Part model, mm, in its own coordinate system. A direction names the side the tool comes from. Give positions to 0.01 mm unless a question says otherwise; leave off trailing zeros. Write each loop counter-clockwise with the first axis right and the second up, starting at its lowest first coordinate (ties: lowest second). Pieces come first, ordered by that corner, then holes. Notation, with made-up numbers: (13.25, -3.5) - (61.25, -3.5) arc R23 ccw to (61.25, 12.5) - close; hole circle Ø5 at (70.5, 10). An arc over 180 degrees is marked (long way). Answer in a Markdown table with one row per item. Add a question column.
1. Which spindle directions (+Z, -Z, +X, -X, +Y, -Y) get a long thin tool onto all of the face, cutting with end or side? Do faces 1 (the flat face through (-1, 20, 14)), 2 (the flat face through (41, 1.75, 18)), 3 (the flat face through (-1, 22.5, 13)). Say none if no direction does.
2. Band-saw the part on B-B on x = 32.25. Write the cut outline in (y, z).
3. Probe line 1 along Y through (x, z) = (-23.5, 9); line 2 along X through (y, z) = (11.5, 20.75); line 3 along Y through (x, z) = (32.25, 1.6). List the from-to ranges inside material, lowest first.
4. Band-saw the part on C-C on y = 0. Write the cut outline in (x, z) (3 decimals).
5. Drop a flat-ended pin along its axis: pin 1 Ø8 at (x, y) = (24, -4) entering from +Z. Give the stop position or say it passes through.
6. Band-saw the part on A-A on z = 18. State how many separate pieces and enclosed holes the cut face has, plus the area to 3 significant figures.
7. Pull direction X, two halves, no side cores. Call faces 4 (the flat face through (-1.75, 21, 18)), 5 (the cylindrical face through (41.9, 21.93, 12.82)), 6 (the flat face through (-42.5, 0, 13)): released by +X, released by -X, zero draft, split by the parting line, or undercut.
8. Band-saw the part on D-D on z = 12. Write the cut outline in (x, y), plus the area to 3 significant figures.
```python
from build123d import *

# Parameters (mm, degrees)
F0_W      = 85
F0_H      = 45
F0_W_2    = 80
F0_H_2    = 40
F1_DEPTH  = 3
F2_DEPTH  = 26
F4_R      = 2.5
F5_DEPTH  = 20
F6_W      = 3.5
F6_H      = 3
F7_DEPTH  = 85.001
F8_W      = 3.5
F8_H      = 3
F9_DEPTH  = 30
F10_R     = 2
F11_R     = 5.75
F12_DEPTH = 3


with BuildPart() as f1:
    # F0 (on Top) → F1 (new body)
    with BuildSketch(Plane.XY):
        Rectangle(F0_W, F0_H)
        Rectangle(F0_W_2, F0_H_2, mode=Mode.SUBTRACT)
        Rectangle(F0_W_2, F0_H_2)
    extrude(amount=F1_DEPTH)

    # F0 (on Top) → F2 (join)
    with BuildSketch(Plane.XY):
        Rectangle(F0_W, F0_H)
        Rectangle(F0_W_2, F0_H_2, mode=Mode.SUBTRACT)
    extrude(amount=F2_DEPTH)

    # F4 (on offset) → F5 (join, through all)
    with BuildSketch(Plane.XY.offset(23)):
        with Locations((-40, 20)):
            Circle(F4_R)
        with Locations((40, 20)):
            Circle(F4_R)
        with Locations((40, -20)):
            Circle(F4_R)
        with Locations((-40, -20)):
            Circle(F4_R)
    extrude(amount=-F5_DEPTH)

    # F6 (on face) → F7 (cut, through all)
    with BuildSketch(Plane(origin=(-42.5, 0, 0), x_dir=(0, -1, 0), z_dir=(-1, 0, 0))):
        with Locations((0, 18.475)):
            Rectangle(F6_W, F6_H)
    extrude(amount=-F7_DEPTH, mode=Mode.SUBTRACT)

    # F8 (on Front) → F9 (cut, symmetric)
    with BuildSketch(Plane.XZ):
        with Locations((0, 18.475)):
            Rectangle(F8_W, F8_H)
    extrude(amount=F9_DEPTH, both=True, mode=Mode.SUBTRACT)

    # F10
    f10_edges = [f1.edges().sort_by_distance(p)[0] for p in [
        (-42.5, -22.5, 13),
        (42.5, -22.5, 13),
        (-42.5, 22.5, 13),
        (42.5, 22.5, 13),
    ]]
    fillet(f10_edges, radius=F10_R)

    # F11 (on face) → F12 (cut, through all)
    with BuildSketch(Plane.XY.offset(3)):
        with Locations((32.25, 0)):
            Circle(F11_R)
    extrude(amount=-F12_DEPTH, mode=Mode.SUBTRACT)


solid = f1.part
```
Values:
| question | item | result |
|---|---|---|
| 1 | face 1 | +Z |
| 1 | face 2 | +X, -X |
| 1 | face 3 | +Z, -Z, +X, -X, +Y |
| 2 | outline | (-22.5, 0) - (-5.75, 0) - (-5.75, 3) - (-20, 3) - (-20, 26) - (-22.5, 26) - close; (5.75, 0) - (22.5, 0) - (22.5, 26) - (20, 26) - (20, 3) - (5.75, 3) - close |
| 3 | line 1 | y = -22.5 to -20, 20 to 22.5 |
| 3 | line 2 | x = -42.5 to -40, 40 to 42.5 |
| 3 | line 3 | y = -22.5 to -5.75, 5.75 to 22.5 |
| 4 | outline | (-42.5, 0) - (26.5, 0) - (26.5, 3) - (-40, 3) - (-40, 16.975) - (-42.5, 16.975) - close; (-42.5, 19.975) - (-40, 19.975) - (-40, 26) - (-42.5, 26) - close; (38, 0) - (42.5, 0) - (42.5, 16.975) - (40, 16.975) - (40, 3) - (38, 3) - close; (40, 19.975) - (42.5, 19.975) - (42.5, 26) - (40, 26) - close |
| 5 | pin 1 | stops at z = 3 |
| 6 | separate pieces | 4 |
| 6 | enclosed holes | 0 |
| 6 | area | 606 mm² |
| 7 | face 4 | undercut |
| 7 | face 5 | released by +X |
| 7 | face 6 | released by -X |
| 8 | outline | (-42.5, -20.5) arc R2 ccw to (-40.5, -22.5) - (40.5, -22.5) arc R2 ccw to (42.5, -20.5) - (42.5, 20.5) arc R2 ccw to (40.5, 22.5) - (-40.5, 22.5) arc R2 ccw to (-42.5, 20.5) - close; hole (-40, -17.5) arc R2.5 cw to (-37.5, -20) - (37.5, -20) arc R2.5 cw to (40, -17.5) - (40, 17.5) arc R2.5 cw to (37.5, 20) - (-37.5, 20) arc R2.5 cw to (-40, 17.5) - close |
| 8 | area | 641 mm² |
